```python
from build123d import *

# Parameters (mm, degrees)
ESQUISSE1_R               = 5
BOSS_EXTRU_1_DEPTH        = 86.4
TROU_TARAUD_M4X0_71_D     = 3.3
TROU_TARAUD_M4X0_71_DEPTH = 20
TROU_TARAUD_M4X0_71_TIP   = 0.991420021
TROU_TARAUD_M4X0_72_D     = 3.3
TROU_TARAUD_M4X0_72_DEPTH = 20
TROU_TARAUD_M4X0_72_TIP   = 0.991420021
CHANFREIN1_SIZE           = 0.5


with BuildPart() as part:
    # Esquisse1 → Boss.-Extru.1 (new body)
    with BuildSketch(Plane.XY):
        Circle(ESQUISSE1_R)
    extrude(amount=BOSS_EXTRU_1_DEPTH)

    # Trou taraudé M4x0.71
    with Locations(Plane.XY.offset(86.4)):
        with Locations((0, 0)):
            Hole(TROU_TARAUD_M4X0_71_D / 2, depth=TROU_TARAUD_M4X0_71_DEPTH)
            with Locations((0, 0, -(TROU_TARAUD_M4X0_71_DEPTH + TROU_TARAUD_M4X0_71_TIP / 2))):  # 118° drill point
                Cone(0, TROU_TARAUD_M4X0_71_D / 2, TROU_TARAUD_M4X0_71_TIP, mode=Mode.SUBTRACT)

    # Trou taraudé M4x0.72
    with Locations(Plane(origin=(0, 0, 0), x_dir=(-1, 0, 0), z_dir=(0, 0, -1))):
        with Locations((0, 0)):
            Hole(TROU_TARAUD_M4X0_72_D / 2, depth=TROU_TARAUD_M4X0_72_DEPTH)
            with Locations((0, 0, -(TROU_TARAUD_M4X0_72_DEPTH + TROU_TARAUD_M4X0_72_TIP / 2))):  # 118° drill point
                Cone(0, TROU_TARAUD_M4X0_72_D / 2, TROU_TARAUD_M4X0_72_TIP, mode=Mode.SUBTRACT)

    # Chanfrein1
    chanfrein1_edges = [part.edges().sort_by_distance(p)[0] for p in [
        (-5, 0, 0),
        (-5, 0, 86.4),
    ]]
    chamfer(chanfrein1_edges, length=CHANFREIN1_SIZE)


solid = part.part
```
Input: part model. Units: mm. Frame: model coordinates. A direction names the side the tool comes from. Coordinates: 2 decimals unless noted, no trailing zeros. Write each loop counter-clockwise with the first axis right and the second up, starting at its lowest first coordinate (ties: lowest second). Pieces come first, ordered by that corner, then holes. Notation, with made-up numbers: (7, 36) -> (65, 36) arc R10 ccw to (65, 44) -> close; hole circle Ø2 at (67.25, -23). An arc over 180 degrees is marked (long way). Write each question's results on one line, items separated by ' | '.
Item 1: Section query A-A on z = 8.5. Return loops of the section in (x, y), plus the area to 3 significant figures.
Conclusion:
outline: circle Ø10 at (0, 0); hole circle Ø3.3 at (0, 0) | area: 70.0 mm^2
Item 2: Set-up query: faces 5 (the flat face through (0, -2, 86.4)), 6 (the cylindrical face through (-1.216, 1.115, 10.14)), 7 (the cylindrical face through (1.216, 1.115, 76.26)). Return all of +Z, -Z, +X, -X, +Y, -Y with unobstructed straight access to the full face (end or side cutting, diameter ignored); none if empty.
Conclusion:
face 5: +Z, +X, -X, +Y, -Y | face 6: -Z | face 7: +Z
Item 3: Material intervals for probe 1 along Y at (x, z) = (0, 4.5); probe 2 along Y at (x, z) = (0.25, 50); probe 3 along X at (y, z) = (-3, 37), sorted ascending.
Conclusion:
probe 1: y = -5 to -1.65, 1.65 to 5 | probe 2: y = -4.99 to 4.99 | probe 3: x = -4 to 4
Item 4: Mould query, pull axis X, two halves, no side actions, for faces 1 (the conical face through (-0.1, -0.3, 65.6)), 2 (the conical face through (-0.3, -0.1, 20.8)), 3 (the flat face through (0, -2, 0)), 4 (the cylindrical face through (-1.08, -4.88, 42.6)). Classes: +X half, -X half, draft (parallel to the pull), parting line (faces both ways), or undercut.
Conclusion:
face 1: undercut | face 2: undercut | face 3: draft | face 4: parting line
Item 5: Section query B-B on z = 50. Return loops of the section in (x, y).
Conclusion:
outline: circle Ø10 at (0, 0)
Item 6: Pin query (flat end, axial travel): pin 1 Ø1 at (x, z) = (-3, 36) entering from -Y; pin 2 Ø5 at (x, z) = (-3, 18) entering from +Y; pin 3 Ø3 at (x, z) = (-2, 41.5) entering from -Y. Return the tip coordinate at first contact, or that it passes through.
Conclusion:
pin 1: stops at y = -4.33 | pin 2: stops at y = 4.97 | pin 3: stops at y = -4.97
